Read the model definition and answer for the solid it produces. Units are mm, in the model's axes. A direction names the side the tool comes from. Give positions to 0.01 mm unless a question says otherwise; leave off trailing zeros. Order: outer loops, then holes, each group sorted by start corner. A loop starts at its lowest first (then second) coordinate and runs counter-clockwise, first axis right, second up. Notation, with made-up numbers: (1.25, -17) - (10.25, -17) arc R21 ccw to (10.25, -3) - close; hole circle Ø11 at (-23.75, 52). An arc over 180 degrees is marked (long way). Return JSON: item names as keys, results as strings.
Autodesk Inventor part; units mm, degrees
ref_plane "YZ Plane" through (0, 0, 0) normal (1, 0, 0) x (0, 1, 0)
ref_plane "XZ Plane" through (0, 0, 0) normal (0, 1, 0) x (-1, 0, 0)
ref_plane "XY Plane" through (0, 0, 0) normal (0, 0, 1) x (1, 0, 0)
sketch "Sketch1" plane through (0, 0, 0) normal (0, 1, 0) x (-1, 0, 0)
  line L0 (19, 19) -> (-19, 19)
  line L1 (-19, 19) -> (-19, -19)
  line L2 (-19, -19) -> (19, -19)
  line L3 (19, -19) -> (19, 19)
  line L4 (19, 19) -> (-19, -19) construction
  line L5 (-19, 19) -> (19, -19) construction
  point P0 (0, 0)
  dimension "d0" = 38
  dimension "d1" = 38
extrude "Extrusion1" add sketch "Sketch1" along normal blind 1.6
sketch "Sketch2" plane through (0, 1.6, 0) normal (0, 1, 0) x (1, 0, 0)
  line L0 (-8.5, -8.5) -> (8.5, -8.5)
  line L1 (8.5, -8.5) -> (8.5, 8.5)
  line L2 (8.5, 8.5) -> (-8.5, 8.5)
  line L3 (-8.5, 8.5) -> (-8.5, -8.5)
  line L4 (-8.5, -8.5) -> (8.5, 8.5) construction
  line L5 (8.5, -8.5) -> (-8.5, 8.5) construction
  circle A0 centre (-8.5, 0) radius 3.5
  circle A1 centre (8.5, 0) radius 3.5
  point P0 (0, 0)
  point P1 (8.5, -3.5)
  point P2 (8.5, 3.5)
  point P3 (-8.5, 3.5)
  point P4 (-8.5, -3.5)
  dimension "d4" = 17
  dimension "d5" = 17
  dimension "d6" = 7
  dimension "d7" = 7
extrude "Extrusion2" add sketch "Sketch2" along normal blind 10.25
sketch "Sketch3" plane through (0, 11.85, 0) normal (0, 1, 0) x (1, 0, 0)
  circle A0 centre (0, 0) radius 7.6
  dimension "d10" = 15.2
extrude "Extrusion3" add sketch "Sketch3" along normal blind 4.31
sketch "Sketch4" plane through (0, 16.16, 0) normal (0, 1, 0) x (1, 0, 0)
  circle A0 centre (0, 0) radius 6.83
  dimension "d13" = 13.66
extrude "Extrusion4" cut sketch "Sketch4" against normal blind 4.31
sketch "Sketch5" plane through (0, 11.85, 0) normal (0, 1, 0) x (1, 0, 0)
  point P0 (0, 0)
properties part number "Camera Top"
Q1. A cutting plane is placed at D-D (x = -15.5). Write down the section's boundary in (y, z).
Values:
{"outline": "(0, -19) - (1.6, -19) - (1.6, 19) - (0, 19) - close"}
Q2. Consider L1, parallel to X at y = 15.2, z = 0; L2, parallel to Y at x = 9, z = 9.5. Determine where each line is inside the solid, lowest interval first.
Values:
{"L1": "x = -7.6 to -6.83, 6.83 to 7.6", "L2": "y = 0 to 1.6"}
Q3. Given pin 1 (8 mm diameter, centred on x = 3, y = 6.5, fed in from -Z); pin 2 (1 mm diameter, centred on y = 3.5, z = 1.5, fed in from -X); pin 3 (10 mm diameter, centred on x = -13.5, z = 3, fed in from +Y), each flat-ended and moving along its own axis, determine where each tip first touches the part or whether it passes through.
Values:
{"pin 1": "stops at z = -8.5", "pin 2": "stops at x = -11.85", "pin 3": "stops at y = 11.85"}
Q4. For faces 5 (the flat face through (-8.5, 7, -6)), 6 (the cylindrical face through (-12, 7, 0)), 7 (the flat face through (8.5, 7, -6)), determine the directions among +Z, -Z, +X, -X, +Y, -Y from which every point of the face is accessible in a straight line to the end or side of a thin tool.
Values:
{"face 5": "-Z, -X, +Y", "face 6": "-X, +Y", "face 7": "-Z, +X, +Y"}
Q5. A cutting plane is placed at C-C (x = 0). Write down the section's boundary in (y, z), and give its area (3 significant figures).
Values:
{"outline": "(0, -19) - (1.6, -19) - (1.6, -8.5) - (11.85, -8.5) - (11.85, -7.6) - (16.16, -7.6) - (16.16, -6.83) - (11.85, -6.83) - (11.85, 6.83) - (16.16, 6.83) - (16.16, 7.6) - (11.85, 7.6) - (11.85, 8.5) - (1.6, 8.5) - (1.6, 19) - (0, 19) - close", "area": "242 mm²"}
Q6. A cutting plane is placed at A-A (z = 0). Write down the section's boundary in (x, y), and give its area (3 significant figures).
Values:
{"outline": "(-19, 0) - (19, 0) - (19, 1.6) - (12, 1.6) - (12, 11.85) - (7.6, 11.85) - (7.6, 16.16) - (6.83, 16.16) - (6.83, 11.85) - (-6.83, 11.85) - (-6.83, 16.16) - (-7.6, 16.16) - (-7.6, 11.85) - (-12, 11.85) - (-12, 1.6) - (-19, 1.6) - close", "area": "313 mm²"}
Q7. Determine the mould class of faces 1 (the flat face through (0, 1.6, 9)), 2 (the flat face through (0, 7, -8.5)), 3 (the flat face through (0, 7, 8.5)), 4 (the flat face through (0, 11.85, 0)) for opening direction Z: released by +Z, released by -Z, zero draft, split by the parting line, or undercut.
Values:
{"face 1": "zero draft", "face 2": "released by -Z", "face 3": "released by +Z", "face 4": "undercut"}
Q8. A cutting plane is placed at B-B (y = 10.25). Write down the section's boundary in (x, z).
Values:
{"outline": "(-8.5, -8.5) - (8.5, -8.5) - (8.5, -3.5) arc R3.5 ccw to (8.5, 3.5) - (8.5, 8.5) - (-8.5, 8.5) - (-8.5, 3.5) arc R3.5 ccw to (-8.5, -3.5) - close"}
